The model under review builds one solid part; all positions refer to its coordinate system, in mm. Face numbers are marked on the shaded views. Round coordinates to 2 decimals unless told otherwise and drop trailing zeros. Loops run counter-clockwise (first coordinate to the right, second up) from the corner with the lowest first, then second, coordinate; pieces in that order, holes last. Notation, with made-up numbers: (-23.75, 31) -> (30.25, 31) arc R22 ccw to (30.25, 45) -> close; hole circle Ø4 at (22, 7). An arc over 180 degrees is marked (long way). Use CSV: the item, a comma, the result in double quotes. Start each with the question number.
```python
from build123d import *

# Parameters (mm, degrees)
SKETCH1_R           = 49.5046
BOSS_EXTRUDE1_DEPTH = 5.08
SKETCH2_R           = 47.625
BOSS_EXTRUDE2_DEPTH = 5.08
SKETCH3_R           = 11.1125
SKETCH3_R_2         = 3.96875
SKETCH3_R_3         = 10
SKETCH3_R_4         = 2
CUT_EXTRUDE1_DEPTH  = 11.16
SKETCH7_R           = 52.166274697
CUT_EXTRUDE4_DEPTH  = 5.08


with BuildPart() as part:
    # Sketch1 → Boss-Extrude1 (new body)
    with BuildSketch(Plane.XY):
        Circle(SKETCH1_R)
    extrude(amount=BOSS_EXTRUDE1_DEPTH)

    # Sketch2 → Boss-Extrude2 (add)
    with BuildSketch(Plane.XY.offset(5.08)):
        Circle(SKETCH2_R)
    extrude(amount=BOSS_EXTRUDE2_DEPTH)

    # Sketch3 → Cut-Extrude1 (cut, through all)
    with BuildSketch(Plane.XY.offset(10.16)):
        with Locations((-12.7, -31.166793627)):
            Circle(SKETCH3_R)
        with Locations((12.7, -31.166793627)):
            Circle(SKETCH3_R)
        with Locations((-36.83, 0)):
            Circle(SKETCH3_R_2)
        with Locations((36.83, 0)):
            Circle(SKETCH3_R_2)
        with Locations((0, 6.35)):
            Circle(SKETCH3_R_3)
        with Locations((0, 28.326878759)):
            Circle(SKETCH3_R_4)
        with Locations((21.976878759, 6.35)):
            Circle(SKETCH3_R_4)
        with Locations((0, -15.626878759)):
            Circle(SKETCH3_R_4)
        with Locations((-21.976878759, 6.35)):
            Circle(SKETCH3_R_4)
        with BuildLine():
            Line((-7.809345457, -12.873575281), (-8.863831528, -12.873575281))
            ThreePointArc((-8.863831528, -12.873575281), (-14.921345457, -17.318575281), (-20.978859386, -12.873575281))
            Line((-20.978859386, -12.873575281), (-22.033345457, -12.873575281))
            ThreePointArc((-22.033345457, -12.873575281), (-23.938345457, -10.968575281), (-22.033345457, -9.063575281))
            Line((-22.033345457, -9.063575281), (-20.978859386, -9.063575281))
            ThreePointArc((-20.978859386, -9.063575281), (-14.921345457, -4.618575281), (-8.863831528, -9.063575281))
            Line((-8.863831528, -9.063575281), (-7.809345457, -9.063575281))
            ThreePointArc((-7.809345457, -9.063575281), (-5.904345457, -10.968575281), (-7.809345457, -12.873575281))
        make_face()
    extrude(amount=-CUT_EXTRUDE1_DEPTH, mode=Mode.SUBTRACT)

    # Sketch7 → Cut-Extrude4 (cut)
    with BuildSketch(Plane(origin=(0, 0, 0), x_dir=(-1, 0, 0), z_dir=(0, 0, -1))):
        Circle(SKETCH7_R)
    extrude(amount=-CUT_EXTRUDE4_DEPTH, mode=Mode.SUBTRACT)


solid = part.part
```
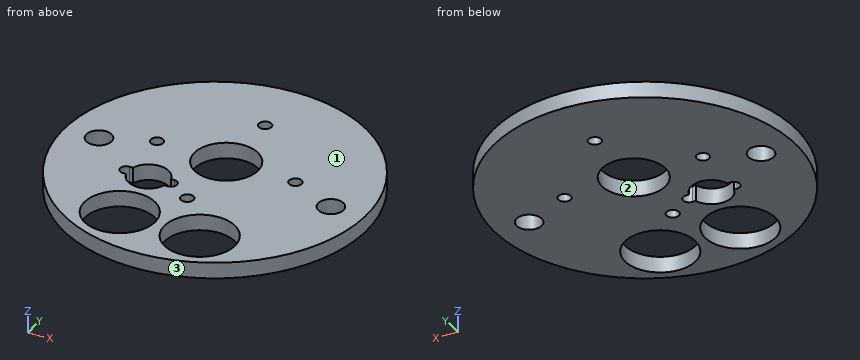
1. Take a section at D-D, the plane x = -12.7. Give the boundary of the cut face in (y, z).
2. Take a section at B-B, the plane z = 7.4. Count the separate pieces of the cut face and the enclosed holes in it, then the cut area to 3 significant figures.
3. Clearance check with flat-ended pins moving along their axes: P1, Ø0.5, axis at x = -8.5, z = 7.5, coming from the -Y side (3 decimals); P2, Ø3, axis at x = -21.98, y = 6.35, coming from the +Z side; P3, Ø1, axis at y = 24, z = 8.5, coming from the +X side; P4, Ø0.5, axis at x = -21.5, z = 7, coming from the +Y side. State where each tip first meets the part, or that it passes through.
4. The part is to be moulded in two halves that separate along Y. For the marked faces 1, 2 and 3, say which applies: pulls with the +Y half, pulls with the -Y half, needs draft (parallel to the pull), parting line crosses it, or undercut.
5. For line 1 along Y through (x, z) = (0, 8.5) (3 decimals); line 2 along Y through (x, z) = (-18, 9.5); line 3 along Y through (x, z) = (-12.7, 7.55), list the stretches that pass through material, from the lowest coordinate up. Write a range as from..to.
6. Take a section at A-A, the plane x = 0. Give the boundary of the cut face in (y, z) (3 decimals), then the cut area to 3 significant figures.
7. Take a section at C-C, the plane y = 6.35. Give the boundary of the cut face in (x, z), then the cut area to 3 significant figures.
Results:
1,outline,"(-45.9, 5.08) -> (-42.28, 5.08) -> (-42.28, 10.16) -> (-45.9, 10.16) -> close; (-20.05, 5.08) -> (-16.92, 5.08) -> (-16.92, 10.16) -> (-20.05, 10.16) -> close; (-5.02, 5.08) -> (45.9, 5.08) -> (45.9, 10.16) -> (-5.02, 10.16) -> close"
2,separate pieces,"1"
2,enclosed holes,"10"
2,area,"5,740 mm²"
3,P1,"y = -46.905"
3,P2,"through"
3,P3,"x = 41.42"
3,P4,"y = 42.62"
4,face 1,"needs draft"
4,face 2,"undercut"
4,face 3,"parting line crosses it"
5,line 1,"-47.625..-17.627, -13.627..-3.65, 16.35..26.327, 30.327..47.625"
5,line 2,"-44.09..-40.93, -21.4..-16.52, -5.41..44.09"
5,line 3,"-45.9..-42.28, -20.05..-16.92, -5.02..45.9"
6,outline,"(-47.625, 5.08) -> (-17.627, 5.08) -> (-17.627, 10.16) -> (-47.625, 10.16) -> close; (-13.627, 5.08) -> (-3.65, 5.08) -> (-3.65, 10.16) -> (-13.627, 10.16) -> close; (16.35, 5.08) -> (26.327, 5.08) -> (26.327, 10.16) -> (16.35, 10.16) -> close; (30.327, 5.08) -> (47.625, 5.08) -> (47.625, 10.16) -> (30.327, 10.16) -> close"
6,area,"342 mm²"
7,outline,"(-47.2, 5.08) -> (-23.98, 5.08) -> (-23.98, 10.16) -> (-47.2, 10.16) -> close; (-19.98, 5.08) -> (-10, 5.08) -> (-10, 10.16) -> (-19.98, 10.16) -> close; (10, 5.08) -> (19.98, 5.08) -> (19.98, 10.16) -> (10, 10.16) -> close; (23.98, 5.08) -> (47.2, 5.08) -> (47.2, 10.16) -> (23.98, 10.16) -> close"
7,area,"337 mm²"
